Read the model definition and answer for the solid it produces. Units are mm, in the model's axes. A direction names the side the tool comes from. Give positions to 0.01 mm unless a question says otherwise; leave off trailing zeros. Order: outer loops, then holes, each group sorted by start corner. A loop starts at its lowest first (then second) coordinate and runs counter-clockwise, first axis right, second up. Notation, with made-up numbers: (83, 39) - (132, 39) arc R20 cw to (132, 43) - close; hole circle Ø3 at (89, 58). An arc over 180 degrees is marked (long way). Use a Markdown table: item, result. Add a question column.
1. Flat-ended cylindrical pins translate along their axes: P1, Ø4.5, axis at y = 20, z = 18, coming from the -X side; P2, Ø4.5, axis at y = 48, z = 18, coming from the +X side; P3, Ø2, axis at y = 17, z = 10.5, coming from the +X side. Find the tip coordinate at first contact, or state that the pin passes through.
2. A cutting plane is placed at C-C on y = 40.5. Determine the outline of the cut face in (x, z), and give its area (3 significant figures).
3. A cutting plane is placed at B-B on x = 5. Determine the outline of the cut face in (y, z), and give its area (3 significant figures).
4. For a pull along X with two mould halves and no side action, classify faces 4 (the conical face through (14.365, 20.323, 17.648)), 5 (the flat face through (5, 0, 5)), 6 (the cylindrical face through (13.642, 50.727, 6.591)) as released by +X, released by -X, zero draft, split by the parting line, or undercut.
5. A cutting plane is placed at A-A on z = 11.5. Determine the outline of the cut face in (x, y).
6. Which of the six approach directions +Z, -Z, +X, -X, +Y, -Y give full straight-line access (tool end or side, diameter ignored) to faces 1 (the flat face through (5, 40, 30)), 2 (the cylindrical face through (6.591, 50.727, 18.358)), 3 (the cylindrical face through (17.642, 22.727, 6.591))?
7. A cutting plane is placed at D-D on z = 23. Determine the outline of the cut face in (x, y).
8. Consider L1, parallel to Y at x = 7, z = 18; L2, parallel to Y at x = 2, z = 15.5; L3, parallel to X at y = 20, z = 5. Determine where each line is inside the solid, lowest interval first.
```python
from build123d import *

# Parameters (mm, degrees)
SCHIZZO1_W                   = 30
SCHIZZO1_H                   = 40
ESTRUSIONE_ESTRUSIONE1_DEPTH = 30
SMUSSO1_SIZE                 = 20
ESTRUSIONE_ESTRUSIONE2_DEPTH = 20
FORO_PER_VITE_M5_1_D         = 5.5
FORO_PER_VITE_M5_1_DEPTH     = 13
FORO_PER_VITE_M5_1_TIP       = 1.652366702
FORO_PER_VITE_M5_2_D         = 5.5
FORO_PER_VITE_M5_2_DEPTH     = 13
FORO_PER_VITE_M5_2_TIP       = 1.652366702


with BuildPart() as part:
    # Schizzo1 → Estrusione-Estrusione1 (new body)
    with BuildSketch(Plane.XY):
        with Locations((15, 20)):
            Rectangle(SCHIZZO1_W, SCHIZZO1_H)
    extrude(amount=ESTRUSIONE_ESTRUSIONE1_DEPTH)

    # Smusso1
    smusso1_edges = [part.edges().sort_by_distance(p)[0] for p in [
        (30, 20, 30),
        (30, 0, 15),
        (15, 0, 30),
    ]]
    chamfer(smusso1_edges, length=SMUSSO1_SIZE)

    # Schizzo2 → Estrusione-Estrusione2 (add)
    with BuildSketch(Plane(origin=(0, 40, 0), x_dir=(1, 0, 0), z_dir=(0, 1, 0))):
        Polygon((0, 0), (30, 0), (30, -10), (10, -30), (0, -30), align=None)
    extrude(amount=ESTRUSIONE_ESTRUSIONE2_DEPTH)

    # Foro per Vite M5-1
    with Locations(Plane.ZY):
        with Locations((18, 20), (18, 48)):
            Hole(FORO_PER_VITE_M5_1_D / 2, depth=FORO_PER_VITE_M5_1_DEPTH)
            with Locations((0, 0, -(FORO_PER_VITE_M5_1_DEPTH + FORO_PER_VITE_M5_1_TIP / 2))):  # 118° drill point
                Cone(0, FORO_PER_VITE_M5_1_D / 2, FORO_PER_VITE_M5_1_TIP, mode=Mode.SUBTRACT)

    # Foro per Vite M5-2
    with Locations(Plane(origin=(18, 20, 0), x_dir=(-1, 0, 0), z_dir=(0, 0, -1))):
        with Locations((0, 0), (4, 28)):
            Hole(FORO_PER_VITE_M5_2_D / 2, depth=FORO_PER_VITE_M5_2_DEPTH)
            with Locations((0, 0, -(FORO_PER_VITE_M5_2_DEPTH + FORO_PER_VITE_M5_2_TIP / 2))):  # 118° drill point
                Cone(0, FORO_PER_VITE_M5_2_D / 2, FORO_PER_VITE_M5_2_TIP, mode=Mode.SUBTRACT)


solid = part.part
```
Output values:
| question | item | result |
|---|---|---|
| 1 | P1 | x = 13.3 |
| 1 | P2 | x = 24.25 |
| 1 | P3 | x = 27.87 |
| 2 | outline | (0, 0) - (30, 0) - (30, 10) - (10, 30) - (0, 30) - close |
| 2 | area | 700 mm² |
| 3 | outline | (0, 0) - (60, 0) - (60, 30) - (20, 30) - (0, 10) - close; hole circle Ø5.5 at (20, 18); hole circle Ø5.5 at (48, 18) |
| 3 | area | 1,550 mm² |
| 4 | face 4 | released by -X |
| 4 | face 5 | zero draft |
| 4 | face 6 | undercut |
| 5 | outline | (0, 1.5) - (10, 1.5) - (28.5, 20) - (28.5, 60) - (0, 60) - close; hole circle Ø5.5 at (14, 48); hole circle Ø5.5 at (18, 20) |
| 6 | face 1 | +Z, +X, -X, +Y, -Y |
| 6 | face 2 | -X |
| 6 | face 3 | -Z |
| 7 | outline | (0, 13) - (10, 13) - (17, 20) - (17, 60) - (0, 60) - close |
| 8 | L1 | 8 to 17.25, 22.75 to 45.25, 50.75 to 60 |
| 8 | L2 | 5.5 to 18.85, 21.15 to 46.85, 49.15 to 60 |
| 8 | L3 | 0 to 15.25, 20.75 to 30 |
